from build123d import *

# Parameters (mm, degrees)
PAD_DEPTH = 6


with BuildPart() as part:
    # Sketch → Pad (new body)
    with BuildSketch(Plane.XZ):
        with BuildLine():
            ThreePointArc((-263.75, 6.3), (-270.05, 0), (-263.75, -6.3))
            Line((263.75, -6.3), (-263.75, -6.3))
            ThreePointArc((263.75, -6.3), (270.05, 0), (263.75, 6.3))
            Line((-263.75, 6.3), (263.75, 6.3))
        make_face()
        with BuildLine():
            ThreePointArc((-263.75, 4.8), (-268.55, 0), (-263.75, -4.8))
            Line((-263.75, -4.8), (263.749984, -4.8))
            ThreePointArc((263.749984, -4.8), (268.55, -8e-06), (263.75, 4.8))
            Line((263.75, 4.8), (-263.75, 4.8))
        make_face(mode=Mode.SUBTRACT)
    extrude(amount=PAD_DEPTH)


solid = part.part
The listing builds one solid part. Answer for the finished solid, in the listing's coordinates (mm). Give positions to 0.01 mm unless a question says otherwise; leave off trailing zeros. Order: outer loops, then holes, each group sorted by start corner. A loop starts at its lowest first (then second) coordinate and runs counter-clockwise, first axis right, second up. Notation, with made-up numbers: (80.5, 32) - (95.5, 32) arc R4 ccw to (95.5, 38) - close; hole circle Ø6 at (-12.5, -3.75). An arc over 180 degrees is marked (long way). One line per item, written item: value. Start each with the question number.
1) Find the intervals of material crossed by L1, parallel to X at y = -4.8, z = -1; L2, parallel to Z at x = 67, y = -5.35; L3, parallel to X at y = -0.3, z = 0, in increasing order.
2) A cutting plane is placed at C-C on z = 0. Give the vertices of the cut face in (x, y), then the cut area to 3 significant figures.
3) A cutting plane is placed at B-B on y = -2.2. Give the vertices of the cut face in (x, z).
4) Given pin 1 Ø1.5 at (y, z) = (-1, 1.5) entering from +X; pin 2 Ø3 at (y, z) = (-3.5, 5) entering from +X, each flat-ended and moving along its own axis, determine where each tip first touches the part or whether it passes through.
5) A cutting plane is placed at A-A on x = -4.5. Give the vertices of the cut face in (y, z).
Answer sheet:
1. L1: x = -269.97 to -268.44, 268.44 to 269.97
1. L2: z = -6.3 to -4.8, 4.8 to 6.3
1. L3: x = -270.05 to -268.55, 268.55 to 270.05
2. outline: (-270.05, -6) - (-268.55, -6) - (-268.55, 0) - (-270.05, 0) - close; (268.55, -6) - (270.05, -6) - (270.05, 0) - (268.55, 0) - close
2. area: 18.0 mm2
3. outline: (-263.75, -6.3) - (263.75, -6.3) arc R6.3 ccw to (263.75, 6.3) - (-263.75, 6.3) arc R6.3 ccw to start; hole (-263.75, -4.8) - (263.75, -4.8) arc R4.8 ccw to (263.75, 4.8) - (-263.75, 4.8) arc R4.8 ccw to start
4. pin 1: stops at x = 270.01
4. pin 2: stops at x = 268.99
5. outline: (-6, -6.3) - (0, -6.3) - (0, -4.8) - (-6, -4.8) - close; (-6, 4.8) - (0, 4.8) - (0, 6.3) - (-6, 6.3) - close
